CAD build for the part. Positions are in the model's coordinates, mm. A direction names the side the tool comes from. Coordinates: 2 decimals unless noted, no trailing zeros. Loops run counter-clockwise (first coordinate to the right, second up) from the corner with the lowest first, then second, coordinate; pieces in that order, holes last.
1) Saw through at C-C, the plane x = 9.5. Write the cut outline in (y, z), and give its area (3 significant figures).
2) Pin check, flat tips, straight feed: pin 1 Ø1.5 at (x, z) = (8.5, 6) entering from +Y; pin 2 Ø3 at (x, z) = (-22.5, 20) entering from +Y. Stop position of each tip, or through.
3) Saw through at B-B, the plane y = 7.75. Write the cut outline in (x, z).
4) Wall check: line 1 along Z through (x, y) = (-0.5, 7); line 2 along X through (y, z) = (1.15, 31.55). Give the ranges that are in metal, low to high.
5) Saw through at D-D, the plane y = 1.25. Write the cut outline in (x, z), and give its area (3 significant figures).
6) Saw through at A-A, the plane z = -22. Write the cut outline in (x, y).
7) Which spindle directions (+Z, -Z, +X, -X, +Y, -Y) get a long thin tool onto all of the face, cutting with end or side? Do faces 3 (the cylindrical face through (19.85, 7.54, -25.6)), 4 (the flat face through (-3, 8, -24.25)), 5 (the cylindrical face through (-26.51, 7.54, -25.53)), 6 (the flat face through (-23, 2, -32)), 7 (the flat face through (-27.866, 3, 0)). Say none if no direction does.
8) Two-plate mould, pull along Z, no slides. Class faces 1 (the flat face through (6, 5, -31)), 2 (the flat face through (-3, 8, -4.85)): +Z half, -Z half, draft (parallel to the pull), parting line (faces both ways), or undercut.
```python
from build123d import *

# Parameters (mm, degrees)
BOSS_EXTRUDE1_DEPTH      = 10
CUT_EXTRUDE3_DEPTH       = 5
BOSS_EXTRUDE6_DEPTH      = 5
BOSS_EXTRUDE6_DEPTH_BACK = 10
SKETCH5_W                = 4.5
SKETCH5_H                = 5
CUT_EXTRUDE5_DEPTH       = 60
CUT_EXTRUDE7_DEPTH       = 5
CUT_EXTRUDE9_DEPTH       = 14
SKETCH9_R                = 2.35
BOSS_EXTRUDE7_DEPTH      = 2
SKETCH12_R               = 2.35
CUT_EXTRUDE10_DEPTH      = 2


with BuildPart() as part:
    # Sketch1 → Boss-Extrude1 (new body)
    with BuildSketch(Plane(origin=(0, 0, 0), x_dir=(1, 0, 0), z_dir=(0, 1, 0))):
        with BuildLine():
            Line((-23.3656, -38.85), (16.6344, -38.85))
            ThreePointArc((16.6344, -38.85), (19.816380515, -37.531980515), (21.1344, -34.35))
            Line((21.1344, -34.35), (21.1344, 34.35))
            ThreePointArc((21.1344, 34.35), (19.816380515, 37.531980515), (16.6344, 38.85))
            Line((16.6344, 38.85), (-23.3656, 38.85))
            ThreePointArc((-23.3656, 38.85), (-26.547580515, 37.531980515), (-27.8656, 34.35))
            Line((-27.8656, 34.35), (-27.8656, -34.35))
            ThreePointArc((-27.8656, -34.35), (-26.547580515, -37.531980515), (-23.3656, -38.85))
        make_face()
    extrude(amount=BOSS_EXTRUDE1_DEPTH)

    # Sketch2 → Cut-Extrude3 (cut)
    with BuildSketch(Plane(origin=(0, 10, 0), x_dir=(1, 0, 0), z_dir=(0, 1, 0))):
        with BuildLine():
            Line((-23.0156, -14.55), (-27.8656, -14.55))
            Line((-27.8656, -14.55), (-27.8656, -28.75))
            ThreePointArc((-27.8656, -28.75), (-26.547580515, -25.568019485), (-23.3656, -24.25))
            Line((-23.3656, -24.25), (16.6344, -24.25))
            ThreePointArc((16.6344, -24.25), (19.816380515, -25.568019485), (21.1344, -28.75))
            Line((21.1344, -28.75), (21.1344, -14.55))
            Line((21.1344, -14.55), (16.2844, -14.55))
            Line((16.2844, -14.55), (-23.0156, -14.55))
        make_face()
        with BuildLine():
            ThreePointArc((-23.0156, -14.55), (-26.445067903, -13.129467874), (-27.8656, -9.699999958))
            Line((-27.8656, -9.699999958), (-27.8656, -14.55))
            Line((-27.8656, -14.55), (-23.0156, -14.55))
        make_face()
        with BuildLine():
            Line((21.1344, -14.55), (21.1344, -9.7))
            ThreePointArc((21.1344, -9.7), (19.713867889, -13.129467889), (16.2844, -14.55))
            Line((16.2844, -14.55), (21.1344, -14.55))
        make_face()
        with BuildLine():
            Line((21.1344, -9.7), (21.1344, -4.85))
            Line((21.1344, -4.85), (16.28440001, -4.85))
            ThreePointArc((16.28440001, -4.85), (19.713867892, -6.270532115), (21.1344, -9.7))
        make_face()
        with BuildLine():
            Line((-23.0156, -4.85), (-27.8656, -4.85))
            Line((-27.8656, -4.85), (-27.8656, -9.699999958))
            ThreePointArc((-27.8656, -9.699999958), (-26.445067874, -6.270532097), (-23.0156, -4.85))
        make_face()
        Polygon((-23.0156, 4.85), (-27.8656, 4.85), (-27.8656, -4.85), (-23.0156, -4.85), (16.28440001, -4.85), (21.1344, -4.85), (21.1344, 4.85), (16.284399974, 4.85), align=None)
        with BuildLine():
            ThreePointArc((-23.0156, 4.85), (-26.445067902, 6.270532124), (-27.8656, 9.700000036))
            Line((-27.8656, 9.700000036), (-27.8656, 4.85))
            Line((-27.8656, 4.85), (-23.0156, 4.85))
        make_face()
        with BuildLine():
            Line((21.1344, 4.85), (21.1344, 9.7))
            ThreePointArc((21.1344, 9.7), (19.71386788, 6.270532102), (16.284399974, 4.85))
            Line((16.284399974, 4.85), (21.1344, 4.85))
        make_face()
        with BuildLine():
            Line((-23.015600011, 14.55), (-27.8656, 14.55))
            Line((-27.8656, 14.55), (-27.8656, 9.700000036))
            ThreePointArc((-27.8656, 9.700000036), (-26.44506788, 13.129467898), (-23.015600011, 14.55))
        make_face()
        with BuildLine():
            Line((16.6344, 24.25), (-23.3656, 24.25))
            ThreePointArc((-23.3656, 24.25), (-26.547580515, 25.568019485), (-27.8656, 28.75))
            Line((-27.8656, 28.75), (-27.8656, 14.55))
            Line((-27.8656, 14.55), (-23.015600011, 14.55))
            Line((-23.015600011, 14.55), (16.2844, 14.55))
            Line((16.2844, 14.55), (21.1344, 14.55))
            Line((21.1344, 14.55), (21.1344, 28.75))
            ThreePointArc((21.1344, 28.75), (19.816380515, 25.568019485), (16.6344, 24.25))
        make_face()
        with BuildLine():
            Line((21.1344, 9.7), (21.1344, 14.55))
            Line((21.1344, 14.55), (16.2844, 14.55))
            ThreePointArc((16.2844, 14.55), (19.713867889, 13.129467889), (21.1344, 9.7))
        make_face()
    extrude(amount=-CUT_EXTRUDE3_DEPTH, mode=Mode.SUBTRACT)

    # Sketch4 → Boss-Extrude6 (add, two sides: drawn at the far end of the back side and taken through both)
    with BuildSketch(Plane.XZ.offset(-BOSS_EXTRUDE6_DEPTH_BACK)):
        with BuildLine():
            ThreePointArc((-27.8656, 34.35), (-26.547580515, 37.531980515), (-23.3656, 38.85))
            Line((-23.3656, 38.85), (-27.8656, 38.85))
            Line((-27.8656, 38.85), (-27.8656, 34.35))
        make_face()
        with BuildLine():
            Line((-23.3656, 35.615611346), (-23.3656, 38.85))
            ThreePointArc((-23.3656, 38.85), (-26.547580515, 37.531980515), (-27.8656, 34.35))
            Line((-27.8656, 34.35), (-27.8656, 34.176611106))
            Line((-27.8656, 34.176611106), (-23.3656, 35.615611346))
        make_face()
        with BuildLine():
            Line((17.428758808, 36.847416441), (16.6344, 38.85))
            ThreePointArc((16.6344, 38.85), (19.816380515, 37.531980515), (21.1344, 34.35))
            Line((21.1344, 34.35), (17.428758808, 36.847416441))
        make_face()
        with BuildLine():
            Line((21.1344, 38.85), (21.1344, 34.35))
            ThreePointArc((21.1344, 34.35), (19.816380515, 37.531980515), (16.6344, 38.85))
            Line((16.6344, 38.85), (21.1344, 38.85))
        make_face()
        with BuildLine():
            Line((16.6344, -34.745010915), (21.1344, -34.35))
            ThreePointArc((21.1344, -34.35), (19.816380515, -37.531980515), (16.6344, -38.85))
            Line((16.6344, -38.85), (16.6344, -34.745010915))
        make_face()
        with BuildLine():
            Line((16.6344, -38.85), (21.1344, -38.85))
            Line((21.1344, -38.85), (21.1344, -34.35))
            ThreePointArc((21.1344, -34.35), (19.816380515, -37.531980515), (16.6344, -38.85))
        make_face()
        with BuildLine():
            Line((-23.3656, -38.85), (-23.156696732, -35.585785164))
            Line((-23.156696732, -35.585785164), (-27.8656, -34.35))
            ThreePointArc((-27.8656, -34.35), (-26.547580515, -37.531980515), (-23.3656, -38.85))
        make_face()
        with BuildLine():
            Line((-27.8656, -34.35), (-27.8656, -38.85))
            Line((-27.8656, -38.85), (-23.3656, -38.85))
            ThreePointArc((-23.3656, -38.85), (-26.547580515, -37.531980515), (-27.8656, -34.35))
        make_face()
    extrude(amount=BOSS_EXTRUDE6_DEPTH + BOSS_EXTRUDE6_DEPTH_BACK)

    # Sketch5 → Cut-Extrude5 (cut)
    with BuildSketch(Plane(origin=(21.1344, 0, 0), x_dir=(0, 0, -1), z_dir=(1, 0, 0))):
        Polygon((34.35, 0), (-34.35, 0), (-34.35, -5), (-38.85, -5), (-38.85, -11.467862175), (41.584838498, -11.467862175), (41.584838498, 0), (38.85, 0), (38.85, -5), (34.35, -5), align=None)
        with Locations((36.6, -2.5)):
            Rectangle(SKETCH5_W, SKETCH5_H)
        with Locations((-36.6, -2.5)):
            Rectangle(SKETCH5_W, SKETCH5_H)
    extrude(amount=-CUT_EXTRUDE5_DEPTH, mode=Mode.SUBTRACT)

    # Sketch6 → Cut-Extrude7 (cut)
    with BuildSketch(Plane.XZ):
        with BuildLine():
            ThreePointArc((-27.8656, 34.05), (-26.45971255, 37.44411255), (-23.0656, 38.85))
            Line((-23.0656, 38.85), (-27.8656, 38.85))
            Line((-27.8656, 38.85), (-27.8656, 34.05))
        make_face()
        with BuildLine():
            Line((-18.2656, 34.05), (-18.2656, 38.85))
            Line((-18.2656, 38.85), (-23.0656, 38.85))
            ThreePointArc((-23.0656, 38.85), (-19.67148745, 37.44411255), (-18.2656, 34.05))
        make_face()
        Polygon((-8.2656, 38.85), (-18.2656, 38.85), (-18.2656, 34.05), (-18.2656, -34.05), (-18.2656, -38.85), (-8.2656, -38.85), (-8.2656, -33.950000026), (-8.2656, 33.95), align=None)
        with BuildLine():
            Line((-3.365599985, 38.85), (-8.2656, 38.85))
            Line((-8.2656, 38.85), (-8.2656, 33.95))
            ThreePointArc((-8.2656, 33.95), (-6.830423222, 37.414823233), (-3.365599985, 38.85))
        make_face()
        with BuildLine():
            Line((1.5344, 38.85), (-3.365599985, 38.85))
            ThreePointArc((-3.365599985, 38.85), (0.099223233, 37.414823222), (1.5344, 33.95))
            Line((1.5344, 33.95), (1.5344, 38.85))
        make_face()
        Polygon((1.5344, 38.85), (1.5344, 33.95), (1.5344, -33.95), (1.5344, -38.85), (11.5344, -38.85), (11.5344, -34.050000018), (11.5344, 34.05), (11.5344, 38.85), align=None)
        with BuildLine():
            Line((16.3344, 38.85), (11.5344, 38.85))
            Line((11.5344, 38.85), (11.5344, 34.05))
            ThreePointArc((11.5344, 34.05), (12.94028745, 37.44411255), (16.3344, 38.85))
        make_face()
        with BuildLine():
            Line((21.1344, 38.85), (16.3344, 38.85))
            ThreePointArc((16.3344, 38.85), (19.72851255, 37.44411255), (21.1344, 34.05))
            Line((21.1344, 34.05), (21.1344, 38.85))
        make_face()
        with BuildLine():
            ThreePointArc((21.1344, -34.05), (19.72851255, -37.44411255), (16.3344, -38.85))
            Line((16.3344, -38.85), (21.1344, -38.85))
            Line((21.1344, -38.85), (21.1344, -34.05))
        make_face()
        with BuildLine():
            Line((11.5344, -34.050000018), (11.5344, -38.85))
            Line((11.5344, -38.85), (16.3344, -38.85))
            ThreePointArc((16.3344, -38.85), (12.940287457, -37.444112556), (11.5344, -34.050000018))
        make_face()
        with BuildLine():
            Line((1.5344, -38.85), (1.5344, -33.95))
            ThreePointArc((1.5344, -33.95), (0.099223245, -37.414823211), (-3.365599951, -38.85))
            Line((-3.365599951, -38.85), (1.5344, -38.85))
        make_face()
        with BuildLine():
            ThreePointArc((-3.365599951, -38.85), (-6.830423201, -37.414823254), (-8.2656, -33.950000026))
            Line((-8.2656, -33.950000026), (-8.2656, -38.85))
            Line((-8.2656, -38.85), (-3.365599951, -38.85))
        make_face()
        with BuildLine():
            Line((-18.2656, -38.85), (-18.2656, -34.05))
            ThreePointArc((-18.2656, -34.05), (-19.67148745, -37.44411255), (-23.0656, -38.85))
            Line((-23.0656, -38.85), (-18.2656, -38.85))
        make_face()
        with BuildLine():
            ThreePointArc((-23.0656, -38.85), (-26.459712556, -37.444112543), (-27.8656, -34.049999982))
            Line((-27.8656, -34.049999982), (-27.8656, -38.85))
            Line((-27.8656, -38.85), (-23.0656, -38.85))
        make_face()
    extrude(amount=-CUT_EXTRUDE7_DEPTH, mode=Mode.SUBTRACT)

    # Sketch8 → Cut-Extrude9 (cut)
    with BuildSketch(Plane.XZ):
        with BuildLine():
            Line((-27.8656, 38.85), (-27.8656, 34.05))
            ThreePointArc((-27.8656, 34.05), (-26.45971255, 37.44411255), (-23.0656, 38.85))
            Line((-23.0656, 38.85), (-27.8656, 38.85))
        make_face()
        with BuildLine():
            Line((21.1344, 34.05), (21.1344, 38.85))
            Line((21.1344, 38.85), (16.3344, 38.85))
            ThreePointArc((16.3344, 38.85), (19.72851255, 37.44411255), (21.1344, 34.05))
        make_face()
        with BuildLine():
            Line((16.3344, -38.85), (21.1344, -38.85))
            Line((21.1344, -38.85), (21.1344, -34.05))
            ThreePointArc((21.1344, -34.05), (19.72851255, -37.44411255), (16.3344, -38.85))
        make_face()
        with BuildLine():
            Line((-27.8656, -34.05), (-27.8656, -38.85))
            Line((-27.8656, -38.85), (-23.0656, -38.85))
            ThreePointArc((-23.0656, -38.85), (-26.45971255, -37.44411255), (-27.8656, -34.05))
        make_face()
    extrude(amount=-CUT_EXTRUDE9_DEPTH, mode=Mode.SUBTRACT)

    # Sketch9 → Boss-Extrude7 (add)
    with BuildSketch(Plane(origin=(0, 10, 0), x_dir=(1, 0, 0), z_dir=(0, 1, 0))):
        with Locations(Location((-22.6506, 31.55, 0), (0, 0, 270))):
            Circle(SKETCH9_R)
        with Locations(Location((15.9194, 31.55, 0), (0, 0, 270))):
            Circle(SKETCH9_R)
        with Locations(Location((-22.6506, -31.55, 0), (0, 0, 270))):
            Circle(SKETCH9_R)
        with Locations(Location((15.9194, -31.55, 0), (0, 0, 270))):
            Circle(SKETCH9_R)
    extrude(amount=BOSS_EXTRUDE7_DEPTH)

    # Sketch12 → Cut-Extrude10 (cut)
    with BuildSketch(Plane.XZ):
        with Locations(Location((15.9194, 31.55, 0), (0, 0, 90))):
            Circle(SKETCH12_R)
        with Locations(Location((-22.6506, -31.55, 0), (0, 0, 90))):
            Circle(SKETCH12_R)
        with Locations(Location((-22.6506, 31.55, 0), (0, 0, 90))):
            Circle(SKETCH12_R)
        with Locations(Location((15.9194, -31.584685618, 0), (0, 0, 270))):
            Circle(SKETCH12_R)
    extrude(amount=-CUT_EXTRUDE10_DEPTH, mode=Mode.SUBTRACT)


solid = part.part
```
Data:
1. outline: (5, -38.85) - (10, -38.85) - (10, -24.25) - (5, -24.25) - close; (5, -14.55) - (10, -14.55) - (10, -4.85) - (5, -4.85) - close; (5, 4.85) - (10, 4.85) - (10, 14.55) - (5, 14.55) - close; (5, 24.25) - (10, 24.25) - (10, 38.85) - (5, 38.85) - close
1. area: 243 mm2
2. pin 1: stops at y = 10
2. pin 2: stops at y = 5
3. outline: (-27.87, -34.05) arc R4.8 ccw to (-23.07, -38.85) - (16.33, -38.85) arc R4.8 ccw to (21.13, -34.05) - (21.13, -28.75) arc R4.5 ccw to (16.63, -24.25) - (-23.37, -24.25) arc R4.5 ccw to (-27.87, -28.75) - close; (-27.87, 28.75) arc R4.5 ccw to (-23.37, 24.25) - (16.63, 24.25) arc R4.5 ccw to (21.13, 28.75) - (21.13, 34.05) arc R4.8 ccw to (16.33, 38.85) - (-23.07, 38.85) arc R4.8 ccw to (-27.87, 34.05) - close; (-23.02, -14.55) - (16.28, -14.55) arc R4.85 ccw to (16.28, -4.85) - (-23.02, -4.85) arc R4.85 ccw to start; (-23.02, 4.85) - (16.28, 4.85) arc R4.85 ccw to (16.28, 14.55) - (-23.02, 14.55) arc R4.85 ccw to start
4. line 1: z = -38.85 to -24.25, -14.55 to -4.85, 4.85 to 14.55, 24.25 to 38.85
4. line 2: x = -27.87 to -25, -20.3 to -18.27, -8.27 to 1.53, 11.53 to 13.57, 18.27 to 21.13
5. outline: (-27.87, -34.05) arc R4.8 ccw to (-18.27, -34.05) - (-18.27, 34.05) arc R4.8 ccw to (-27.87, 34.05) - close; (-8.27, -33.95) arc R4.9 ccw to (1.53, -33.95) - (1.53, 33.95) arc R4.9 ccw to (-8.27, 33.95) - close; (11.53, -34.05) arc R4.8 ccw to (21.13, -34.05) - (21.13, 34.05) arc R4.8 ccw to (11.53, 34.05) - close; hole circle Ø4.7 at (-22.65, -31.55); hole circle Ø4.7 at (-22.65, 31.55); hole circle Ø4.7 at (15.92, -31.58); hole circle Ø4.7 at (15.92, 31.55)
5. area: 2,120 mm2
6. outline: (-27.87, 0) - (-18.27, 0) - (-18.27, 5) - (-27.87, 5) - close; (-8.27, 0) - (1.53, 0) - (1.53, 5) - (-8.27, 5) - close; (11.53, 0) - (21.13, 0) - (21.13, 5) - (11.53, 5) - close
7. face 3: +X, +Y
7. face 4: +X, -X, +Y
7. face 5: -X, +Y
7. face 6: -Y
7. face 7: +Z, -Z, -X, +Y, -Y
8. face 1: draft
8. face 2: undercut
